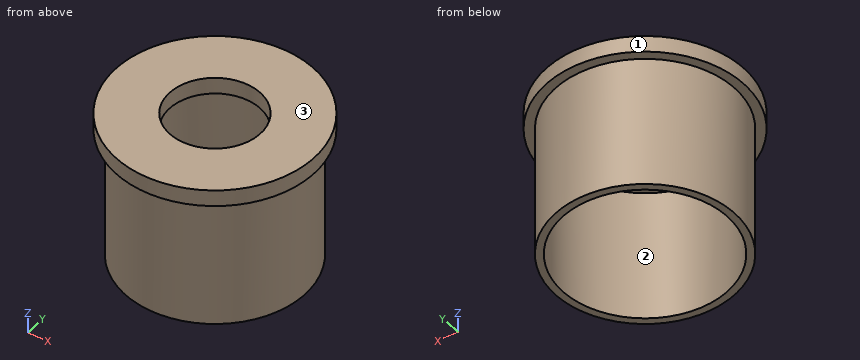
Autodesk Inventor part; units mm, degrees
ref_plane "YZ Plane" through (0, 0, 0) normal (1, 0, 0) x (0, 1, 0)
ref_plane "XZ Plane" through (0, 0, 0) normal (0, 1, 0) x (-1, 0, 0)
ref_plane "XY Plane" through (0, 0, 0) normal (0, 0, 1) x (1, 0, 0)
sketch "Sketch1" plane through (0, 0, 0) normal (0, 0, 1) x (1, 0, 0)
  circle A0 centre (0, 0) radius 17.272
  circle A1 centre (0, 0) radius 19.05
  circle A2 centre (0, 0) radius 15.875
  dimension "d0" = 34.544
  dimension "d1" = 38.1
  dimension "d6" = 31.75
extrude "Extrusion1" add sketch "Sketch1" along normal blind 3.175 contours A0 | A1 | A2
extrude "Extrusion2" add sketch "Sketch1" against normal blind 25.4 contours A0
sketch "Sketch2" plane through (0, 0, 3.175) normal (0, 0, 1) x (1, 0, 0)
  circle A0 centre (0, 0) radius 19.05
  circle A1 centre (0, 0) radius 8.7313
  dimension "d7" = 17.4625
extrude "Extrusion3" cut sketch "Sketch2" against normal blind 25.4 contours A1
properties part number "PVC Cap" material "PVC-Piping"
Verification items for the finished model (mm, model axes). Face numbers are marked on the shaded views. Give positions to 0.01 mm unless a question says otherwise; leave off trailing zeros. Loops run counter-clockwise (first coordinate to the right, second up) from the corner with the lowest first, then second, coordinate; pieces in that order, holes last.
1. Release check for a two-part mould opening along X. For the marked faces 1, 2 and 3 record: +X half, -X half, draft (parallel to the pull), parting line (faces both ways), or undercut.
Derived:
face 1: parting line
face 2: undercut
face 3: draft
2. Cross-section at A-A on y = 0. Record the cut outline in (x, z) (3 decimals), and give its area (3 significant figures).
Derived:
outline: (-19.05, 0) - (-17.272, 0) - (-17.272, -25.4) - (-15.875, -25.4) - (-15.875, 0) - (-8.731, 0) - (-8.731, 3.175) - (-19.05, 3.175) - close; (8.731, 0) - (15.875, 0) - (15.875, -25.4) - (17.272, -25.4) - (17.272, 0) - (19.05, 0) - (19.05, 3.175) - (8.731, 3.175) - close
area: 136 mm2
3. Cross-section at D-D on z = -22.5. Record the cut outline in (x, y) (3 decimals).
Derived:
outline: circle Ø34.544 at (0, 0); hole circle Ø31.75 at (0, 0)
4. Cross-section at C-C on x = -15. Record the cut outline in (y, z) (3 decimals), and give its area (3 significant figures).
Derived:
outline: (-11.743, 0) - (-8.563, 0) - (-8.563, -25.4) - (-5.198, -25.4) - (-5.198, 0) - (5.198, 0) - (5.198, -25.4) - (8.563, -25.4) - (8.563, 0) - (11.743, 0) - (11.743, 3.175) - (-11.743, 3.175) - close
area: 246 mm2
5. Go/stop test with flat-tipped pins: P1, Ø11.5, axis at x = -4, y = -0.5, coming from the -Z side; P2, Ø2, axis at y = -9, z = -19, coming from the -X side; P3, Ø8, axis at x = 0.5, z = 0, coming from the +Y side. Record where each tip stops, or that it passes through.
Derived:
P1: stops at z = 0
P2: stops at x = -15.31
P3: stops at y = 19.05
6. Material ranges on probe 1 along Y at (x, z) = (0, -17) (3 decimals); probe 2 along Z at (x, y) = (11, 2.5) (3 decimals); probe 3 along Y at (x, z) = (0, 1.95), recorded low to high.
Derived:
probe 1: y = -17.272 to -15.875, 15.875 to 17.272
probe 2: z = 0 to 3.175
probe 3: y = -19.05 to -8.73, 8.73 to 19.05
